Build history of the part. All positions in model axes, mm. A direction names the side the tool comes from. Coordinates: 2 decimals unless noted, no trailing zeros. Order: outer loops, then holes, each group sorted by start corner. A loop starts at its lowest first (then second) coordinate and runs counter-clockwise, first axis right, second up. Notation, with made-up numbers: M -33.75,-30 L -18.75,-30 A29 ccw -18.75,-10 Z; hole C 76.5,73.5 d2. An arc over 180 degrees is marked long. Use a Markdown table: item, result. Add a question column.
from build123d import *

# Parameters (mm, degrees)
SKETCH_1_R          = 1.7
EXTRUDE_2_DEPTH     = 3
SKETCH_2_W          = 3
SKETCH_2_H          = 42
EXTRUDE_3_DEPTH     = 19
SKETCH_3_R          = 1.7
CUT_EXTRUDE_1_DEPTH = 5
CUT_EXTRUDE_2_DEPTH = 5
CHAMFER_1_SIZE      = 1


with BuildPart() as part:
    # Эскиз1 → Бобышка-Вытянуть2 (new body)
    with BuildSketch(Plane(origin=(0, 0, 0), x_dir=(0, 0, -1), z_dir=(1, 0, 0))):
        Polygon((0, 38.5), (-5, 38.5), (-5, -3.5), (7.246656809, -3.5), (7.246656809, 38.5), align=None)
        Circle(SKETCH_1_R, mode=Mode.SUBTRACT)
        with BuildLine():
            ThreePointArc((0, 32.3), (-1.7, 34), (0, 35.7))
            ThreePointArc((0, 35.7), (1.7, 34), (0, 32.3))
        make_face(mode=Mode.SUBTRACT)
    extrude(amount=EXTRUDE_2_DEPTH)

    # Эскиз2 → Бобышка-Вытянуть3 (add)
    with BuildSketch(Plane.ZY):
        with Locations((-5.746656809, 17.5)):
            Rectangle(SKETCH_2_W, SKETCH_2_H)
    extrude(amount=EXTRUDE_3_DEPTH)

    # Эскиз3 → Вырез-Вытянуть1 (cut)
    with BuildSketch(Plane.XY.offset(-4.246656809)):
        with Locations((-16, 35.010378706)):
            Circle(SKETCH_3_R)
        with Locations((-16, 1.010378706)):
            Circle(SKETCH_3_R)
    extrude(amount=-CUT_EXTRUDE_1_DEPTH, mode=Mode.SUBTRACT)

    # Эскиз4 → Вырез-Вытянуть2 (cut)
    with BuildSketch(Plane.XY.offset(-4.246656809)):
        with BuildLine():
            Line((-3.030961954, 29.041213722), (-3.030961954, 7.066639766))
            ThreePointArc((-3.030961954, 7.066639766), (-8.041074018, 2.056527703), (-13.051186081, 7.066639766))
            Line((-13.051186081, 7.066639766), (-13.051186081, 29.041213722))
            ThreePointArc((-13.051186081, 29.041213722), (-8.041074018, 34.051325785), (-3.030961954, 29.041213722))
        make_face()
    extrude(amount=-CUT_EXTRUDE_2_DEPTH, mode=Mode.SUBTRACT)

    # Фаска1
    chamfer_1_edges = [part.edges().sort_by_distance(p)[0] for p in [
        (0, 35.7, 0),
        (0, 0, 1.7),
    ]]
    chamfer(chamfer_1_edges, length=CHAMFER_1_SIZE)


solid = part.part
(1) Slice it at D-D on x = -7. Give the cut face in (y, z), and give its area (3 significant figures).
(2) Slice it at B-B on z = 0. Give the cut face in (x, y), and give its area (3 significant figures).
(3) Which spindle directions (+Z, -Z, +X, -X, +Y, -Y) get a long thin tool onto all of the face, cutting with end or side? Do faces 5 (the flat face through (0, 18, 0)), 6 (the flat face through (-6, -3.5, -5)), 7 (the cylindrical face through (-8.15, 34.05, -5.73)). Say none if no direction does.
(4) Drill centre lines: line 1 along Y through (x, z) = (-16, -6.15); line 2 along Y through (x, z) = (1.5, 0); line 3 along Z through (x, y) = (2.65, 34). Where is each one in solid material? Low to high. Write a range as from..to.
(5) Slice it at C-C on x = -16. Give the cut face in (y, z), and give its area (3 significant figures).
(6) Mould opens along Z. For faces 1 (the cylindrical face through (1.99, 32.3, -0.07)), 2 (the flat face through (-6, 38.5, -5)), 3 (the flat face through (-1, 17, -7.247)), 4 (the cylindrical face through (1.99, -1.66, 0.37)) say: released by +Z, released by -Z, zero draft, split by the parting line, or undercut.
(7) Drop flat-ended pins along their axis: P1, Ø1, axis at y = 31, z = 3, coming from the -X side; P2, Ø4.5, axis at y = 0, z = 0, coming from the -X side. Give the stop position or say it passes through.
(8) Slice it at A-A on y = 8. Give the cut face in (x, z).
Solutions:
| question | item | result |
|---|---|---|
| 1 | outline | M -3.5,-7.25 L 2.17,-7.25 L 2.17,-4.25 L -3.5,-4.25 Z; M 33.94,-7.25 L 38.5,-7.25 L 38.5,-4.25 L 33.94,-4.25 Z |
| 1 | area | 30.7 mm² |
| 2 | outline | M 0,-3.5 L 3,-3.5 L 3,-1.7 L 1,-1.7 L 0,-2.7 Z; M 0,2.7 L 1,1.7 L 3,1.7 L 3,32.3 L 1,32.3 L 0,31.3 Z; M 0,36.7 L 1,35.7 L 3,35.7 L 3,38.5 L 0,38.5 Z |
| 2 | area | 104 mm² |
| 3 | face 5 | +Z, -X, +Y, -Y |
| 3 | face 6 | +Z, -Z, +X, -X, -Y |
| 3 | face 7 | +Z, -Z |
| 4 | line 1 | -3.5..-0.69, 2.71..33.31, 36.71..38.5 |
| 4 | line 2 | -3.5..-1.7, 1.7..32.3, 35.7..38.5 |
| 4 | line 3 | -7.25..-1.7, 1.7..5 |
| 5 | outline | M -3.5,-7.25 L -0.69,-7.25 L -0.69,-4.25 L -3.5,-4.25 Z; M 2.71,-7.25 L 33.31,-7.25 L 33.31,-4.25 L 2.71,-4.25 Z; M 36.71,-7.25 L 38.5,-7.25 L 38.5,-4.25 L 36.71,-4.25 Z |
| 5 | area | 106 mm² |
| 6 | face 1 | undercut |
| 6 | face 2 | zero draft |
| 6 | face 3 | released by -Z |
| 6 | face 4 | undercut |
| 7 | P1 | x = 0 |
| 7 | P2 | x = 0.45 |
| 8 | outline | M -19,-7.25 L -13.05,-7.25 L -13.05,-4.25 L -19,-4.25 Z; M -3.03,-7.25 L 3,-7.25 L 3,5 L 0,5 L 0,-4.25 L -3.03,-4.25 Z |
